Can you work these out from the drawing? Everything is in mm from the part's minimum corner. Coordinates: 2 decimals unless noted, no trailing zeros. Order: outer loops, then holes, each group sorted by start corner. A loop starts at its lowest first (then second) coordinate and runs counter-clockwise, first axis right, second up. Notation, with made-up numbers: (-20.5, -22) - (33.5, -22) arc R12 ccw to (33.5, -9) - close; hole circle Ø9 at (62, 74). An arc over 180 degrees is marked (long way). Use a Markdown table: item, result. Add a question column.
(1) If I drill on L1, parallel to Z at x = 69.5, y = 3.4; L2, parallel to X at y = 2.7, z = 8; L3, parallel to X at y = 0.7, z = 156.5, over which ranges is the centre line in solid material (lowest first)? Write a range as [from, to].
(2) I want a section at C-C (z = 15). List the corners of the cut face in (x, y) for me.
(3) I want a section at D-D (x = 71). List the corners of the cut face in (y, z) for me.
(4) For pin 1 Ø2 at (y, z) = (1.5, 2) entering from +X; pin 2 Ø2 at (y, z) = (2.5, 83) entering from -X; pin 3 Ø1.2 at (y, z) = (1.5, 85.5) entering from +X, each with a flat end and sliding along its axis, tell me the tip position at first contact or that it passes through.
(5) I want a section at A-A (x = 131.5). List the corners of the cut face in (y, z) for me, and give its area (3 significant figures).
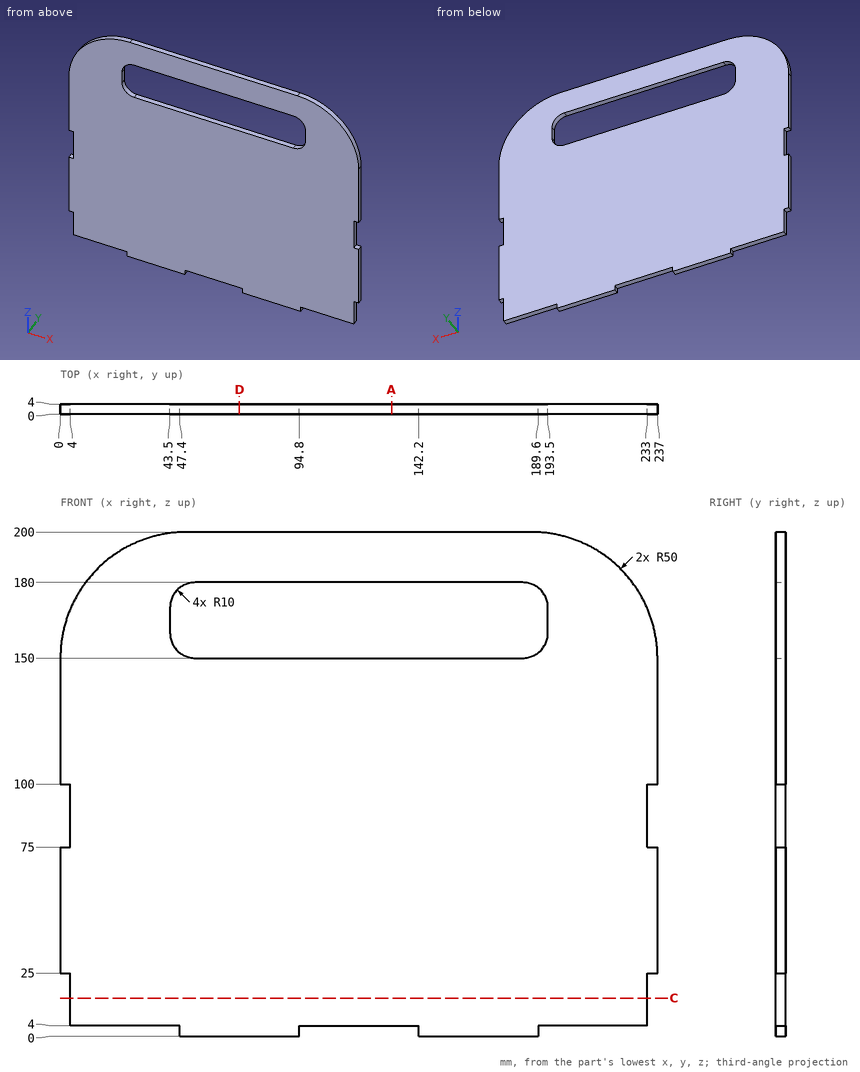
Answers follow:
| question | item | result |
|---|---|---|
| 1 | L1 | z = [0, 150], [180, 200] |
| 1 | L2 | x = [4, 233] |
| 1 | L3 | x = [0.42, 44.13], [192.87, 236.58] |
| 2 | outline | (4, 0) - (233, 0) - (233, 4) - (4, 4) - close |
| 3 | outline | (0, 0) - (4, 0) - (4, 150) - (0, 150) - close; (0, 180) - (4, 180) - (4, 200) - (0, 200) - close |
| 4 | pin 1 | stops at x = 189.6 |
| 4 | pin 2 | stops at x = 4 |
| 4 | pin 3 | stops at x = 233 |
| 5 | outline | (0, 4) - (4, 4) - (4, 150) - (0, 150) - close; (0, 180) - (4, 180) - (4, 200) - (0, 200) - close |
| 5 | area | 664 mm² |
